For this review, use the dimensioned drawing (mm, ordinates from the lowest corner) and the shaded views. A direction names the side the tool comes from. Coordinates: 2 decimals unless noted, no trailing zeros. Loops run counter-clockwise (first coordinate to the right, second up) from the corner with the lowest first, then second, coordinate; pieces in that order, holes last. Notation, with made-up numbers: (57.5, 27.25) -> (92.5, 27.25) arc R17 ccw to (92.5, 44.25) -> close; hole circle Ø5 at (-21, 2.5). An arc over 180 degrees is marked (long way). Answer as a JSON object with one key per item and string values.
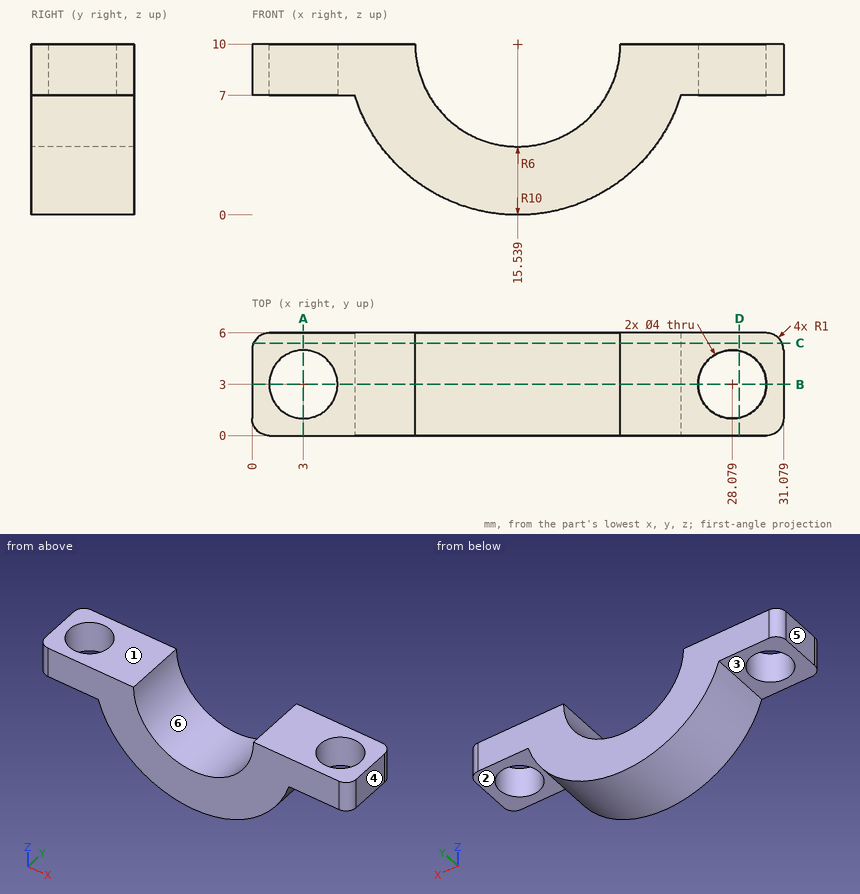
1) Add section A-A, the plane x = 3. Give the boundary of the cut face in (y, z).
Completed:
{"outline": "(0, 7) -> (1, 7) -> (1, 10) -> (0, 10) -> close; (5, 7) -> (6, 7) -> (6, 10) -> (5, 10) -> close"}
2) Add section B-B, the plane y = 3. Give the boundary of the cut face in (x, z).
Completed:
{"outline": "(0, 7) -> (1, 7) -> (1, 10) -> (0, 10) -> close; (5, 7) -> (6, 7) arc R10 ccw to (25.08, 7) -> (26.08, 7) -> (26.08, 10) -> (21.54, 10) arc R6 cw to (9.54, 10) -> (5, 10) -> close; (30.08, 7) -> (31.08, 7) -> (31.08, 10) -> (30.08, 10) -> close"}
3) The part is to be moulded in two halves that separate along X. For the marked faces 4, 5 and 6, say which applies: pulls with the +X half, pulls with the -X half, needs draft (parallel to the pull), parting line crosses it, or undercut.
Completed:
{"face 4": "pulls with the +X half", "face 5": "pulls with the -X half", "face 6": "undercut"}
4) Clearance check with flat-ended pins moving along their axes: pin 1 Ø3 at (y, z) = (3, 2.5) entering from -X; pin 2 Ø1 at (x, y) = (18, 5) entering from -Z; pin 3 Ø2 at (x, y) = (26.5, 3) entering from -Z. State where each tip first meets the part, or that it passes through.
Completed:
{"pin 1": "x = 7.54", "pin 2": "z = 0.19", "pin 3": "z = 7"}
5) Wall thickness on probe 1 along Y at (x, z) = (3, 8.15); probe 2 along Z at (x, y) = (5, 0.9); probe 3 along X at (y, z) = (2.45, 6.5) (1 decimal): over which ranges is each line inside the solid? List them lowest first.
Completed:
{"probe 1": "0 to 1, 5 to 6", "probe 2": "7 to 10", "probe 3": "6.2 to 10.7, 20.4 to 24.9"}
6) Add section C-C, the plane y = 5.4. Give the boundary of the cut face in (x, z) (1 decimal), and give its area (3 significant figures).
Completed:
{"outline": "(0.1, 7) -> (6, 7) arc R10 ccw to (25.1, 7) -> (31, 7) -> (31, 10) -> (21.5, 10) arc R6 cw to (9.5, 10) -> (0.1, 10) -> close", "area": "134 mm²"}
7) For the marked faces 1, 2 and 3, list the 3-axis set-ups (+Z, -Z, +X, -X, +Y, -Y) from which the entire face can be reached by the end or side of a thin tool; tool diameter is ignored.
Completed:
{"face 1": "+Z, +X, -X, +Y, -Y", "face 2": "-Z, +X, +Y, -Y", "face 3": "-Z, -X, +Y, -Y"}
